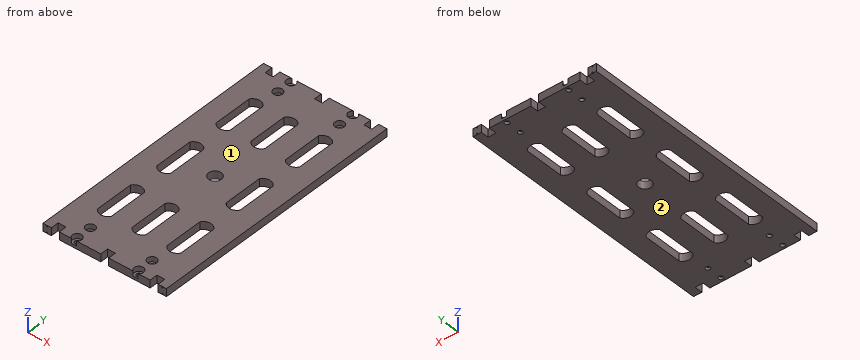
Autodesk Fusion 360 part; units mm, degrees
sketch "Schizzo5" plane through (0, 0, 0) normal (0, 0, 1) x (1, 0, 0)
  line L0 (65.1728, 106.4816) -> (65.1728, -60.7184)
  circle A0 centre (85.1728, -58.2184) radius 1.5
  circle A1 centre (125.1728, 103.9816) radius 3
  line L1 (65.1728, 22.8816) -> (145.1728, 22.8816) construction
  circle A2 centre (85.1728, 103.9816) radius 3
  circle A3 centre (85.1728, 103.9816) radius 1.5
  line L2 (145.1728, 106.4816) -> (65.1728, 106.4816)
  circle A4 centre (125.1728, 103.9816) radius 1.5
  line L3 (105.1728, 25.3816) -> (105.1728, 1.3102) construction
  circle A5 centre (105.1728, 22.8816) radius 4.1
  line L4 (145.1728, -60.7184) -> (145.1728, 106.4816)
  line L5 (85.1728, 106.4816) -> (85.1728, -60.7184) construction
  circle A6 centre (85.1728, -58.2184) radius 3
  circle A7 centre (125.1728, -58.2184) radius 1.5
  line L6 (65.1728, -60.7184) -> (145.1728, -60.7184)
  circle A8 centre (125.1728, -58.2184) radius 3
  line L7 (65.1728, -58.2184) -> (145.1728, -58.2184) construction
  line L8 (105.1728, 106.4816) -> (105.1728, -60.7184) construction
  line L9 (105.1728, 25.3816) -> (105.1728, 56.9762) construction
  line L10 (105.1728, 25.3816) -> (105.1728, 56.9762) construction
  line L11 (105.1728, 25.3816) -> (105.1728, 1.3102) construction
  line L12 (65.1728, -48.2184) -> (145.1728, -48.2184) construction
  circle A9 centre (85.1728, -48.2184) radius 1.5
  circle A10 centre (85.1728, -48.2184) radius 3
  circle A11 centre (125.1728, -48.2184) radius 3
  circle A12 centre (125.1728, -48.2184) radius 1.5
  circle A13 centre (85.1728, 93.9816) radius 3
  circle A14 centre (85.1728, 93.9816) radius 1.5
  circle A15 centre (125.1728, 93.9816) radius 3
  circle A16 centre (125.1728, 93.9816) radius 1.5
  line L13 (107.7228, -60.7184) -> (102.6228, -60.7184)
  line L14 (102.6228, -60.7184) -> (102.6228, -55.6184)
  line L15 (102.6228, -55.6184) -> (107.7228, -55.6184)
  line L16 (107.7228, -55.6184) -> (107.7228, -60.7184)
  line L17 (107.7228, -60.7184) -> (102.6228, -55.6184) construction
  line L18 (102.6228, -60.7184) -> (107.7228, -55.6184) construction
  line L19 (102.6228, 101.3816) -> (107.7228, 101.3816)
  line L20 (102.6228, 106.4816) -> (102.6228, 101.3816)
  line L21 (107.7228, 101.3816) -> (107.7228, 106.4816)
  line L22 (70.6228, -55.6184) -> (75.7228, -55.6184)
  line L23 (75.7228, -55.6184) -> (75.7228, -60.7184)
  line L24 (75.7228, -60.7184) -> (70.6228, -60.7184)
  line L25 (70.6228, -60.7184) -> (70.6228, -55.6184)
  line L26 (134.6228, -55.6184) -> (134.6228, -60.7184)
  line L27 (139.7228, -55.6184) -> (134.6228, -55.6184)
  line L28 (139.7228, -60.7184) -> (139.7228, -55.6184)
  line L29 (134.6228, -60.7184) -> (139.7228, -60.7184)
  line L30 (70.6228, -60.7184) -> (75.7228, -55.6184) construction
  line L31 (70.6228, -55.6184) -> (75.7228, -60.7184) construction
  line L32 (70.6228, 101.3816) -> (75.7228, 101.3816)
  line L33 (75.7228, 101.3816) -> (75.7228, 106.4816)
  line L34 (70.6228, 106.4816) -> (70.6228, 101.3816)
  line L35 (75.7228, 106.4816) -> (70.6228, 106.4816)
  line L36 (139.7228, 101.3816) -> (134.6228, 101.3816)
  line L37 (134.6228, 101.3816) -> (134.6228, 106.4816)
  line L38 (139.7228, 106.4816) -> (139.7228, 101.3816)
  line L39 (134.6228, 106.4816) -> (139.7228, 106.4816)
  line L40 (78.1728, 35.3816) -> (87.1728, 35.3816)
  line L41 (87.1728, 35.3816) -> (87.1728, 10.3816)
  line L42 (87.1728, 10.3816) -> (78.1728, 10.3816)
  line L43 (78.1728, 10.3816) -> (78.1728, 35.3816)
  arc A17 (78.1728, 10.3816) -> (87.1728, 10.3816) centre (82.6728, 13.1816) ccw
  line L44 (78.1728, 22.8816) -> (87.1728, 22.8816) construction
  arc A18 (87.1728, 35.3816) -> (78.1728, 35.3816) centre (82.6728, 32.5816) ccw
  arc A19 (132.1728, 35.3816) -> (123.1728, 35.3816) centre (127.6728, 32.5816) ccw
  line L45 (132.1728, 35.3816) -> (123.1728, 35.3816)
  line L46 (123.1728, 35.3816) -> (123.1728, 10.3816)
  line L47 (132.1728, 10.3816) -> (132.1728, 35.3816)
  line L48 (123.1728, 10.3816) -> (132.1728, 10.3816)
  arc A20 (123.1728, 10.3816) -> (132.1728, 10.3816) centre (127.6728, 13.1816) ccw
  line L49 (82.6728, 35.3816) -> (82.6728, 10.3816) construction
  line L50 (127.6728, 35.3816) -> (127.6728, 10.3816) construction
  line L51 (132.1728, 22.8816) -> (123.1728, 22.8816) construction
  line L52 (109.6728, -34.6184) -> (100.6728, -34.6184)
  line L53 (100.6728, -34.6184) -> (100.6728, -9.6184)
  line L54 (100.6728, -9.6184) -> (109.6728, -9.6184)
  line L55 (109.6728, -9.6184) -> (109.6728, -34.6184)
  line L56 (109.6728, -34.6184) -> (100.6728, -9.6184) construction
  line L57 (100.6728, -34.6184) -> (109.6728, -9.6184) construction
  arc A21 (109.6728, -9.6184) -> (100.6728, -9.6184) centre (105.1728, -12.4184) ccw
  line L58 (100.6728, -22.1184) -> (109.6728, -22.1184) construction
  arc A22 (100.6728, -34.6184) -> (109.6728, -34.6184) centre (105.1728, -31.8184) ccw
  line L59 (82.6728, 37.8816) -> (82.6728, 35.3816) construction
  arc A23 (100.6728, 55.3816) -> (109.6728, 55.3816) centre (105.1728, 58.1816) ccw
  line L60 (109.6728, 55.3816) -> (109.6728, 80.3816)
  line L61 (100.6728, 80.3816) -> (100.6728, 55.3816)
  arc A24 (109.6728, 80.3816) -> (100.6728, 80.3816) centre (105.1728, 77.5816) ccw
  line L62 (100.6728, 80.3816) -> (109.6728, 55.3816) construction
  line L63 (109.6728, 80.3816) -> (100.6728, 55.3816) construction
  line L64 (78.1728, -9.6184) -> (87.1728, -9.6184)
  line L65 (87.1728, -9.6184) -> (87.1728, -34.6184)
  line L66 (87.1728, -34.6184) -> (78.1728, -34.6184)
  line L67 (78.1728, -34.6184) -> (78.1728, -9.6184)
  line L68 (82.6728, -9.6184) -> (82.6728, -34.6184) construction
  line L69 (78.1728, -22.1184) -> (87.1728, -22.1184) construction
  line L70 (82.6728, -9.6184) -> (82.6728, -7.1184) construction
  arc A25 (87.1728, -9.6184) -> (78.1728, -9.6184) centre (82.6728, -12.4184) ccw
  arc A26 (78.1728, -34.6184) -> (87.1728, -34.6184) centre (82.6728, -31.8184) ccw
  arc A27 (132.1728, -9.6184) -> (123.1728, -9.6184) centre (127.6728, -12.4184) ccw
  line L71 (132.1728, -34.6184) -> (132.1728, -9.6184)
  line L72 (123.1728, -9.6184) -> (123.1728, -34.6184)
  arc A28 (123.1728, -34.6184) -> (132.1728, -34.6184) centre (127.6728, -31.8184) ccw
  line L73 (82.6728, 13.1816) -> (82.6728, -60.7184) construction
  arc A29 (78.1728, 55.3816) -> (87.1728, 55.3816) centre (82.6728, 58.1816) ccw
  line L74 (78.1728, 80.3816) -> (78.1728, 55.3816)
  line L75 (87.1728, 55.3816) -> (87.1728, 80.3816)
  arc A30 (87.1728, 80.3816) -> (78.1728, 80.3816) centre (82.6728, 77.5816) ccw
  arc A31 (132.1728, 80.3816) -> (123.1728, 80.3816) centre (127.6728, 77.5816) ccw
  line L76 (132.1728, 80.3816) -> (132.1728, 55.3816)
  line L77 (123.1728, 55.3816) -> (123.1728, 80.3816)
  arc A32 (123.1728, 55.3816) -> (132.1728, 55.3816) centre (127.6728, 58.1816) ccw
  point P0 (105.1728, -58.1684)
  point P1 (105.1728, 25.3816)
  point P2 (73.1728, -58.1684)
  point P3 (82.6728, 22.8816)
  point P4 (127.6728, 22.8816)
  point P5 (105.1728, -22.1184)
  point P6 (105.1728, -7.1184)
  point P7 (105.1728, 67.8816)
  dimension "d221" = 80
  dimension "d222" = 167.2
  dimension "d223" = 2.5
  dimension "d224" = 20
  dimension "d225" = 3
  dimension "d226" = 6
  dimension "d229" = 8.2
  dimension "d350" = 3
  dimension "d351" = 6
  dimension "d354" = 10
  dimension "d355" = 5.1
  dimension "d356" = 5.1
  dimension "d368" = 5.1
  dimension "d369" = 5.1
  dimension "d370" = 32
  dimension "d371" = 9
  dimension "d372" = 25
  dimension "d373" = 45
  dimension "d380" = 9
  dimension "d381" = 25
  dimension "d382" = 2.5
  dimension "d383" = 2.5
  dimension "d384" = 90
  dimension "d385" = 9
  dimension "d386" = 25
  dimension "d387" = 2.5
extrude "Estrusione24" add sketch "Schizzo5" along normal blind 5 contours L0 A1 A2 L2 L4 A6 L6 A8 L14 L15 L16 L19 L20 L21 L22 L23 L25 L26 L27 L28 L32 L33 L34 L36 L37 L38
extrude "Estrusione25" add sketch "Schizzo5" along normal blind 1.8 contours A2 L2 | A6 L6 | A1 L2 | L6 A8 | A10 | A11 | A13 | A15 picked at (85.2101, 106.1469) picked at (85.2101, -60.3837) picked at (125.2101, 106.1469) picked at (125.2101, -60.3837)
sketch "Schizzo17" plane through (0, -60.7184, 0) normal (0, -1, 0) x (1, 0, 0)
  line L0 (75.7228, 0) -> (102.6228, 0)
  line L1 (102.6228, 0) -> (102.6228, 5)
  line L2 (102.6228, 5) -> (86.8311, 5)
  line L3 (86.8311, 5) -> (86.8311, 1.8)
  line L4 (86.8311, 1.8) -> (83.5144, 1.8)
  line L5 (83.5144, 1.8) -> (83.5144, 5)
  line L6 (65.1728, 5) -> (145.1728, 5) construction
  line L7 (145.1728, 5) -> (145.1728, 0) construction
  line L8 (145.1728, 0) -> (65.1728, 0) construction
  line L9 (65.1728, 0) -> (65.1728, 5) construction
  line L10 (107.7228, 0) -> (134.6228, 0) construction
  line L11 (107.7228, 5) -> (123.5144, 5) construction
  line L12 (145.1728, 0) -> (145.1728, 5) construction
  line L13 (65.1728, 2.5) -> (145.1728, 2.5) construction
  line L14 (77.9024, 5) -> (-23.8923, 0) construction
  circle A0 centre (67.723, 4.5) radius 0.4
  circle A1 centre (67.723, 0.5) radius 0.4
  line L15 (105.1728, 5) -> (105.1728, 0) construction
  line L16 (132.4431, 5) -> (234.2378, 0) construction
  circle A2 centre (142.6225, 0.5) radius 0.4
  circle A3 centre (142.6225, 4.5) radius 0.4
  line L17 (83.5144, 5) -> (75.7228, 5)
  line L18 (75.7228, 5) -> (75.7228, 0)
  line L19 (139.7228, 0) -> (145.1728, 0)
  point P0 (142.6225, 4.5)
  point P1 (142.6225, 0.5)
  point P2 (142.6225, 4.5)
  dimension "d357" = 0.8
  dimension "d358" = 4
extrude "Estrusione29" cut sketch "Schizzo17" against normal blind 180 contours A0 | A1 | A2 | A3
equation "d225 = d227"
equation "d226 = d228"
equation "d350 = d227"
equation "d351 = d228"
equation "d355 = d356"
equation "d368 = d356"
equation "d369 = d356"
Work out the finished part from the listing and answer in its coordinate system (mm). Face numbers are marked on the shaded views. Give positions to 0.01 mm unless a question says otherwise; leave off trailing zeros. Order: outer loops, then holes, each group sorted by start corner. A loop starts at its lowest first (then second) coordinate and runs counter-clockwise, first axis right, second up. Notation, with made-up numbers: M -8,-21 L 32,-21 A24 ccw 32,3 Z; hole C -33,6 d6. An arc over 180 degrees is marked long. Return JSON: item names as keys, results as strings.
1) Section B-B, the plane z = 2.65 is taken. Give the number of separate pieces and of enclosed holes in the cut face, plus the area to 3 significant figures.
Resolved:
{"separate pieces": "1", "enclosed holes": "13", "area": "10,900 mm^2"}
2) Straight lines are drawn through the part: line 1 along X through (y, z) = (-15, 4.65); line 2 along X through (y, z) = (18.5, 2.4); line 3 along X through (y, z) = (55.5, 2.1). For each, find the intervals that lie inside material, in ascending order. Write a range as [from, to].
Resolved:
{"line 1": "[65.17, 67.35], [68.09, 78.17], [87.17, 100.67], [109.67, 123.17], [132.17, 142.25], [142.99, 145.17]", "line 2": "[65.17, 78.17], [87.17, 123.17], [132.17, 145.17]", "line 3": "[65.17, 78.17], [87.17, 100.67], [109.67, 123.17], [132.17, 145.17]"}
3) For a pull along Z with two mould halves and no side action, classify the marked faces 1 and 2 as +Z half, -Z half, draft (parallel to the pull), parting line (faces both ways), or undercut.
Resolved:
{"face 1": "+Z half", "face 2": "-Z half"}
4) Each of these flat-tipped pins is pushed along its axis until it touches: pin 1 (1.5 mm diameter, centred on x = 136.5, z = 1.5, fed in from +Y); pin 2 (5 mm diameter, centred on x = 85.17, y = -58.22, fed in from +Z). Where does it stop, or does it pass through?
Resolved:
{"pin 1": "y = 101.38", "pin 2": "z = 1.8"}
5) Section A-A, the plane x = 138 is taken. Write down the section's boundary in (y, z), plus the area to 3 significant figures.
Resolved:
{"outline": "M -55.62,0 L 101.38,0 L 101.38,5 L -55.62,5 Z", "area": "785 mm^2"}
